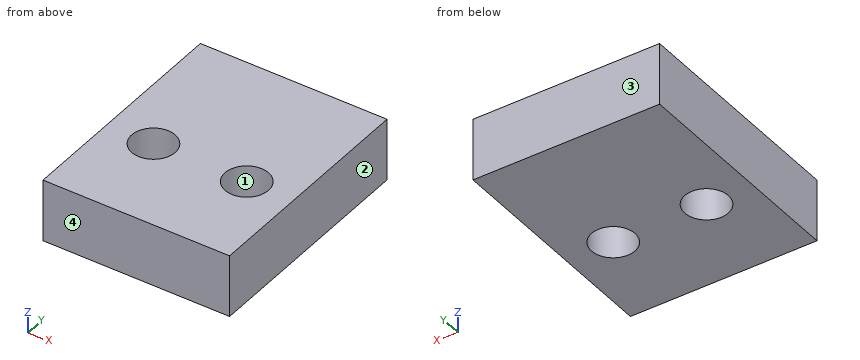
from build123d import *

# Parameters (mm, degrees)
F0_W     = 76.2
F0_H     = 76.2
F0_R     = 8.89
F0_H_2   = 17.78
F1_DEPTH = 25.4


with BuildPart() as f1:
    # F0 (on Top) → F1 (new body)
    with BuildSketch(Plane.XY):
        with Locations((-3.790651, -18.235706)):
            Rectangle(F0_W, F0_H)
        with Locations((-22.840651, -18.235706)):
            Circle(F0_R, mode=Mode.SUBTRACT)
        with Locations((15.259349, -18.235706)):
            Circle(F0_R, mode=Mode.SUBTRACT)
        with Locations((-3.790651, 28.754294)):
            Rectangle(F0_W, F0_H_2)
    extrude(amount=F1_DEPTH)


solid = f1.part
For this review, take the finished solid that the model builds, in its own axes (mm). Face numbers are marked on the shaded views. Give positions to 0.01 mm unless a question says otherwise; leave off trailing zeros. Order: outer loops, then holes, each group sorted by start corner. A loop starts at its lowest first (then second) coordinate and runs counter-clockwise, first axis right, second up. Notation, with made-up numbers: M 28,14 L 35,14 A22 ccw 35,40 Z; hole C 62,8 d4. An arc over 180 degrees is marked long. Answer in a Markdown table with one row per item. Add a question column.
(1) Consider section A-A on x = 11. State the section outline as (y, z) points.
(2) Wall thickness on probe 1 along X at (y, z) = (-21, 8.75); probe 2 along Y at (x, z) = (18.5, 3.5); probe 3 along Y at (x, z) = (-22.5, 23.75): over which ranges is each line inside the solid? List them lowest first. Write a range as [from, to].
(3) Consider section D-D on x = 21. State the section outline as (y, z) points.
(4) Consider section C-C on z = 4.25. State the section outline as (x, y) points, and give its area (3 significant figures).
(5) Consider section B-B on y = -16.5. State the section outline as (x, z) points, and give its area (3 significant figures).
(6) Mouldability with a two-part tool opening along Y and no side actions: class the marked faces 1, 2, 3 and 4 as +Y half, -Y half, draft (parallel to the pull), parting line (faces both ways), or undercut.
(7) For pin 1 (23 mm diameter, centred on x = -22.84, y = -18.24, fed in from +Z), flat-tipped, find the tip position at first contact; note if it passes through.
Evaluation:
| question | item | result |
|---|---|---|
| 1 | outline | M -56.34,0 L -26.04,0 L -26.04,25.4 L -56.34,25.4 Z; M -10.43,0 L 37.64,0 L 37.64,25.4 L -10.43,25.4 Z |
| 2 | probe 1 | x = [-41.89, -31.29], [-14.39, 6.81], [23.71, 34.31] |
| 2 | probe 2 | y = [-56.34, -26.51], [-9.96, 37.64] |
| 2 | probe 3 | y = [-56.34, -27.12], [-9.35, 37.64] |
| 3 | outline | M -56.34,0 L -25.02,0 L -25.02,25.4 L -56.34,25.4 Z; M -11.45,0 L 37.64,0 L 37.64,25.4 L -11.45,25.4 Z |
| 4 | outline | M -41.89,-56.34 L 34.31,-56.34 L 34.31,37.64 L -41.89,37.64 Z; hole C -22.84,-18.24 d17.78; hole C 15.26,-18.24 d17.78 |
| 4 | area | 6,660 mm^2 |
| 5 | outline | M -41.89,0 L -31.56,0 L -31.56,25.4 L -41.89,25.4 Z; M -14.12,0 L 6.54,0 L 6.54,25.4 L -14.12,25.4 Z; M 23.98,0 L 34.31,0 L 34.31,25.4 L 23.98,25.4 Z |
| 5 | area | 1,050 mm^2 |
| 6 | face 1 | undercut |
| 6 | face 2 | draft |
| 6 | face 3 | +Y half |
| 6 | face 4 | -Y half |
| 7 | pin 1 | stops at z = 25.4 |
